```python
from build123d import *

# Parameters (mm, degrees)
SALIENTE_EXTRUIR1_DEPTH    = 1.9
CROQUIS3_R                 = 11.5
CROQUIS3_R_2               = 14
CORTAR_EXTRUIR1_DEPTH      = 1
CORTAR_EXTRUIR1_DEPTH_BACK = 2.9


with BuildPart() as part:
    # Croquis2 → Saliente-Extruir1 (new body)
    with BuildSketch(Plane(origin=(0, 0, 0), x_dir=(1, 0, 0), z_dir=(0, 1, 0))):
        Polygon((438.1, 0), (-438.1, 0), (-438.1, 1000), (-338.1, 1810), (438.1, 1810), align=None)
    extrude(amount=SALIENTE_EXTRUIR1_DEPTH)

    # Croquis3 → Cortar-Extruir1 (cut, two sides)
    with BuildSketch(Plane(origin=(0, 1.9, 0), x_dir=(1, 0, 0), z_dir=(0, 1, 0))) as cortar_extruir1_sk:
        with Locations((338.1, 50)):
            Circle(CROQUIS3_R)
        with Locations((288.1, 50)):
            Circle(CROQUIS3_R_2)
    extrude(amount=CORTAR_EXTRUIR1_DEPTH, mode=Mode.SUBTRACT)
    extrude(cortar_extruir1_sk.sketch, amount=-CORTAR_EXTRUIR1_DEPTH_BACK, mode=Mode.SUBTRACT)


solid = part.part
```
For this review, take the finished solid that the model builds, in its own axes (mm). Round coordinates to 2 decimals unless told otherwise and drop trailing zeros. Order: outer loops, then holes, each group sorted by start corner. A loop starts at its lowest first (then second) coordinate and runs counter-clockwise, first axis right, second up.
Q1. We need section B-B, the plane z = -1495. Give the boundary of the cut face in (x, y), plus the area to 3 significant figures.
Findings below:
outline: (-376.99, 0) - (438.1, 0) - (438.1, 1.9) - (-376.99, 1.9) - close
area: 1,550 mm2
Q2. We need section A-A, the plane y = 1.5. Give the boundary of the cut face in (x, z), plus the area to 3 significant figures.
Findings below:
outline: (-438.1, -1000) - (-338.1, -1810) - (438.1, -1810) - (438.1, 0) - (-438.1, 0) - close; hole circle Ø28 at (288.1, -50); hole circle Ø23 at (338.1, -50)
area: 1,540,000 mm2
Q3. Wall thickness on line 1 (X direction, y = 1, z = -50); line 2 (Z direction, x = 288.1, y = 1.05); line 3 (Z direction, x = 338.1, y = 1.25): over which ranges is each line inside the solid? List them lowest first.
Findings below:
line 1: x = -438.1 to 274.1, 302.1 to 326.6, 349.6 to 438.1
line 2: z = -1810 to -64, -36 to 0
line 3: z = -1810 to -61.5, -38.5 to 0
